Here's how the part is built. I have some questions about the finished solid (model axes, mm). Coordinates: 2 decimals unless noted, no trailing zeros. Write each loop counter-clockwise with the first axis right and the second up, starting at its lowest first coordinate (ties: lowest second). Pieces come first, ordered by that corner, then holes.
from build123d import *

# Parameters (mm, degrees)
SKETCH_1_W          = 50
SKETCH_1_H          = 50
EXTRUDE_1_DEPTH     = 20
CUT_EXTRUDE_1_DEPTH = 20


with BuildPart() as part:
    # Эскиз1 → Бобышка-Вытянуть1 (new body)
    with BuildSketch(Plane(origin=(0, 0, 0), x_dir=(1, 0, 0), z_dir=(0, 1, 0))):
        Rectangle(SKETCH_1_W, SKETCH_1_H)
    extrude(amount=EXTRUDE_1_DEPTH)

    # Эскиз2 → Вырез-Вытянуть1 (cut)
    with BuildSketch(Plane(origin=(0, 20, 0), x_dir=(1, 0, 0), z_dir=(0, 1, 0))):
        Polygon((-0.8, 3.2), (0.8, 3.2), (0.8, -3.2), (0, -3.2), (-0.8, -3.2), align=None)
        Polygon((4.614359354, -16.5), (7.814359354, -10.957437416), (9.2, -11.757437416), (6, -17.3), align=None)
        Polygon((-6, -17.3), (-4.614359354, -16.5), (-7.814359354, -10.957437416), (-9.2, -11.757437416), align=None)
    extrude(amount=-CUT_EXTRUDE_1_DEPTH, mode=Mode.SUBTRACT)


solid = part.part
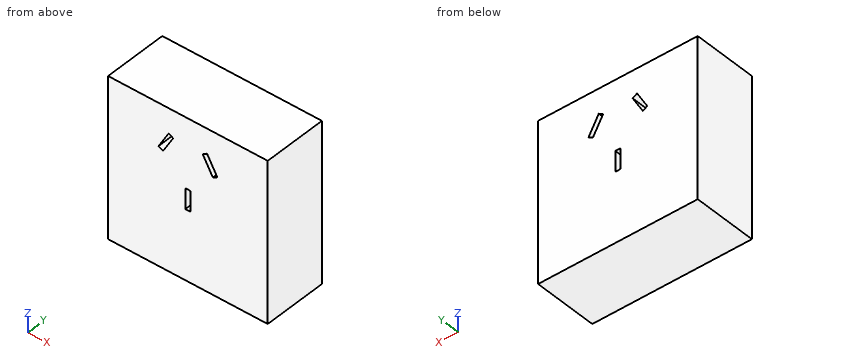
1. For pin 1 Ø5 at (x, z) = (-19.5, -4.5) entering from -Y, with a flat end and sliding along its axis, tell me the tip position at first contact or that it passes through.
2. If I drill on line 1 (X direction, y = 16.75, z = 1); line 2 (Z direction, x = 7, y = 1.25); line 3 (Z direction, x = 8, y = 5.75), over which ranges is the centre line in solid material (lowest first)?
3. I want a section at B-B (z = 14). List the corners of the cut face in (x, y) for me, then the cut area to 3 significant figures.
4. I want a section at A-A (z = 1.5). List the corners of the cut face in (x, y) for me, then the cut area to 3 significant figures.
Response values:
1. pin 1: stops at y = 0
2. line 1: x = -25 to -0.8, 0.8 to 25
2. line 2: z = -25 to 12.37, 15.57 to 25
2. line 3: z = -25 to 11.06, 13.84 to 25
3. outline: (-25, 0) - (-7.91, 0) - (-7.91, 20) - (-25, 20) - close; (-6.06, 0) - (6.06, 0) - (6.06, 20) - (-6.06, 20) - close; (7.91, 0) - (25, 0) - (25, 20) - (7.91, 20) - close
3. area: 926 mm2
4. outline: (-25, 0) - (-0.8, 0) - (-0.8, 20) - (-25, 20) - close; (0.8, 0) - (25, 0) - (25, 20) - (0.8, 20) - close
4. area: 968 mm2
